from build123d import *

# Parameters (mm, degrees)
F0_W     = 150
F0_H     = 15
F0_R     = 3
F1_DEPTH = 1
F2_R     = 7.49999


# Not quite as in the source:
# - a fillet or chamfer is up to 0.001 mm smaller than in the source, because OpenCascade refuses the exact size


with BuildPart() as f1:
    # F0 (on Front) → F1 (new body, symmetric)
    with BuildSketch(Plane.XZ):
        with Locations((67.5, 0)):
            Rectangle(F0_W, F0_H)
        Circle(F0_R, mode=Mode.SUBTRACT)
        with Locations((67.5, 0)):
            Circle(F0_R, mode=Mode.SUBTRACT)
        with Locations((135, 0)):
            Circle(F0_R, mode=Mode.SUBTRACT)
    extrude(amount=F1_DEPTH, both=True)

    # F2 (radius 7.5 in the source; OpenCascade refuses exactly that, so slightly less here)
    f2_edges = [f1.edges().sort_by_distance(p)[0] for p in [
        (142.5, 0, 7.5),
        (142.5, 0, -7.5),
        (-7.5, 0, 7.5),
        (-7.5, 0, -7.5),
    ]]
    fillet(f2_edges, radius=F2_R)


solid = f1.part
Source: CAD feature listing. Evaluate the final solid. Frame: model axes, mm. Coordinates: 2 decimals unless noted, no trailing zeros. Order: outer loops, then holes, each group sorted by start corner. A loop starts at its lowest first (then second) coordinate and runs counter-clockwise, first axis right, second up.
Item 1: Cut plane C-C (z = -1.5). Return loops of the section in (x, y), plus the area to 3 significant figures.
Output values:
outline: (-7.35, -1) - (-2.6, -1) - (-2.6, 1) - (-7.35, 1) - close; (2.6, -1) - (64.9, -1) - (64.9, 1) - (2.6, 1) - close; (70.1, -1) - (132.4, -1) - (132.4, 1) - (70.1, 1) - close; (137.6, -1) - (142.35, -1) - (142.35, 1) - (137.6, 1) - close
area: 268 mm2
Item 2: Pull-direction query (Z, two-part tool) for faces 1 (the face through (66, -1, 3)), 2 (the face through (140.361, -0.014, -5.245)), 3 (the face through (137.86, 0.01, 0.9)); classes: pulls with the +Z half, pulls with the -Z half, needs draft (parallel to the pull), parting line crosses it, or undercut.
Output values:
face 1: needs draft
face 2: pulls with the -Z half
face 3: undercut
Item 3: First-contact query: P1, Ø5, axis at x = 135, z = 0, coming from the -Y side; P2, Ø8, axis at x = 0, z = 0, coming from the -Y side. Flat tips, straight axial feed; report the tip coordinate or a pass-through.
Output values:
P1: passes through
P2: stops at y = -1
Item 4: Cut plane B-B (y = 0.25). Count the separate pieces of the cut face and the enclosed holes in it, plus the area to 3 significant figures.
Output values:
separate pieces: 1
enclosed holes: 3
area: 2,120 mm2
Item 5: Material intervals for line 1 (X direction, y = -0.6, z = -2.25); line 2 (Z direction, x = 67.5, y = -0.5); line 3 (X direction, y = -0.15, z = -1), sorted ascending.
Output values:
line 1: x = -7.15 to -1.98, 1.98 to 65.52, 69.48 to 133.02, 136.98 to 142.15
line 2: z = -7.5 to -3, 3 to 7.5
line 3: x = -7.43 to -2.83, 2.83 to 64.67, 70.33 to 132.17, 137.83 to 142.43
Item 6: Cut plane A-A (x = 67.5). Return loops of the section in (y, z).
Output values:
outline: (-1, -7.5) - (1, -7.5) - (1, -3) - (-1, -3) - close; (-1, 3) - (1, 3) - (1, 7.5) - (-1, 7.5) - close
